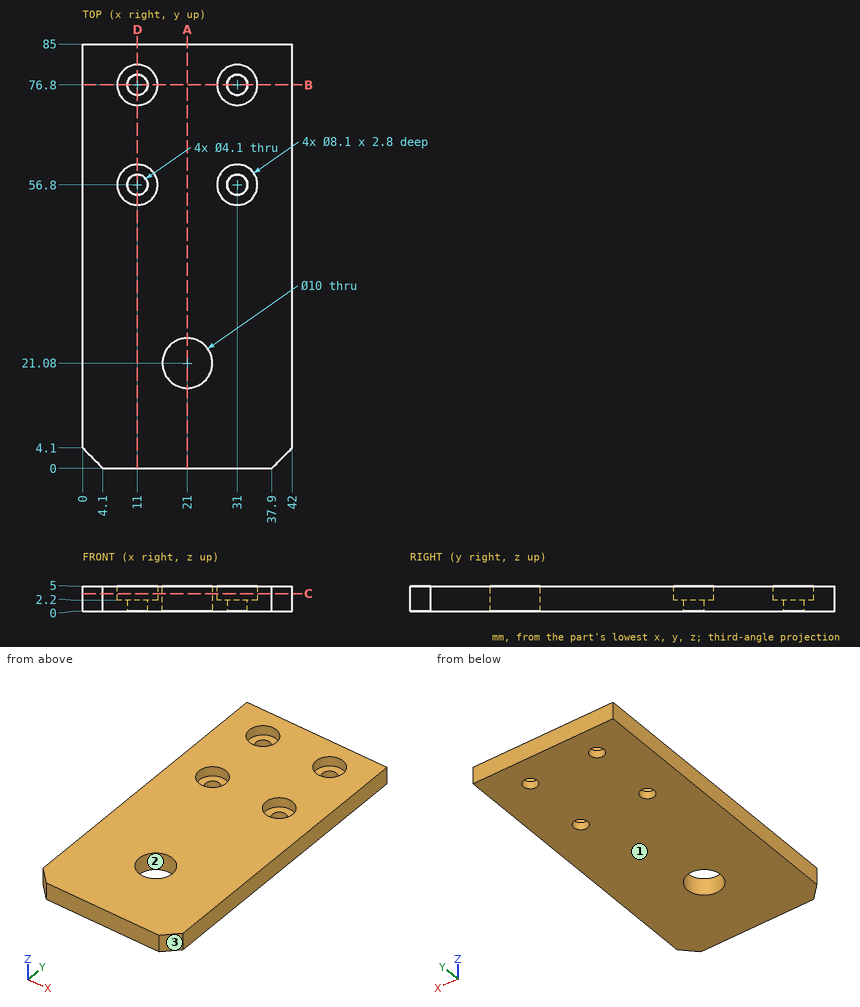
Can you work these out from the drawing? Everything is in mm from the part's minimum corner. Round coordinates to 2 decimals unless told otherwise and drop trailing zeros. Loops run counter-clockwise (first coordinate to the right, second up) from the corner with the lowest first, then second, coordinate; pieces in that order, holes last. Notation, with made-up numbers: (80.5, 39.25) - (89.5, 39.25) arc R10 ccw to (89.5, 44.25) - close; hole circle Ø8 at (42.5, 69). An arc over 180 degrees is marked (long way). Answer in a Markdown table with one row per item. Add a question column.
(1) If we section it at B-B (y = 76.8): Please give me the cut outline in (x, z).
(2) I need wall thicknesses on line 1 along Y through (x, z) = (11, 0.65); line 2 along Y through (x, z) = (11, 4.3); line 3 along X through (y, z) = (56.8, 1.75). Which ranges of each line are inside material? Lowest first, please.
(3) If we section it at D-D (x = 11): Please give me the cut outline in (y, z).
(4) If we section it at A-A (x = 21): Please give me the cut outline in (y, z), plus the area to 3 significant figures.
(5) If we mould it in two halves opening along Y, with no side actions, what happens to the marked faces 1, 2 and 3? For each: pulls with the +Y half, pulls with the -Y half, needs draft (parallel to the pull), parting line crosses it, or undercut.
(6) I'm going to push a flat-ended pin straight in: pin 1 (2.5 mm diameter, centred on x = 10, y = 75, fed in from +Z). Where does the tip first touch, or does it pass through?
(7) If we section it at C-C (z = 3.55): Please give me the cut outline in (x, y), plus the area to 3 significant figures.
Model answer:
| question | item | result |
|---|---|---|
| 1 | outline | (0, 0) - (8.95, 0) - (8.95, 2.2) - (6.95, 2.2) - (6.95, 5) - (0, 5) - close; (13.05, 0) - (28.95, 0) - (28.95, 2.2) - (26.95, 2.2) - (26.95, 5) - (15.05, 5) - (15.05, 2.2) - (13.05, 2.2) - close; (33.05, 0) - (42, 0) - (42, 5) - (35.05, 5) - (35.05, 2.2) - (33.05, 2.2) - close |
| 2 | line 1 | y = 0 to 54.75, 58.85 to 74.75, 78.85 to 85 |
| 2 | line 2 | y = 0 to 52.75, 60.85 to 72.75, 80.85 to 85 |
| 2 | line 3 | x = 0 to 8.95, 13.05 to 28.95, 33.05 to 42 |
| 3 | outline | (0, 0) - (54.75, 0) - (54.75, 2.2) - (52.75, 2.2) - (52.75, 5) - (0, 5) - close; (58.85, 0) - (74.75, 0) - (74.75, 2.2) - (72.75, 2.2) - (72.75, 5) - (60.85, 5) - (60.85, 2.2) - (58.85, 2.2) - close; (78.85, 0) - (85, 0) - (85, 5) - (80.85, 5) - (80.85, 2.2) - (78.85, 2.2) - close |
| 4 | outline | (0, 0) - (16.08, 0) - (16.08, 5) - (0, 5) - close; (26.08, 0) - (85, 0) - (85, 5) - (26.08, 5) - close |
| 4 | area | 375 mm² |
| 5 | face 1 | needs draft |
| 5 | face 2 | undercut |
| 5 | face 3 | pulls with the -Y half |
| 6 | pin 1 | stops at z = 2.2 |
| 7 | outline | (0, 4.1) - (4.1, 0) - (37.9, 0) - (42, 4.1) - (42, 85) - (0, 85) - close; hole circle Ø8.1 at (11, 56.8); hole circle Ø8.1 at (11, 76.8); hole circle Ø10 at (21, 21.08); hole circle Ø8.1 at (31, 56.8); hole circle Ø8.1 at (31, 76.8) |
| 7 | area | 3,270 mm² |
